CAD build for the part. Positions are in the model's coordinates, mm. A direction names the side the tool comes from. Give positions to 0.01 mm unless a question says otherwise; leave off trailing zeros. Write each loop counter-clockwise with the first axis right and the second up, starting at its lowest first coordinate (ties: lowest second). Pieces come first, ordered by that corner, then holes. Notation, with made-up numbers: (65, -25) -> (105, -25) arc R20 ccw to (105, -11) -> close; hole circle Ø3 at (-7.75, -15.75). An arc over 180 degrees is marked (long way). Answer as a JSON object with one key per item and string values.
```python
from build123d import *

# Parameters (mm, degrees)
SKETCH1_W                     = 30
SKETCH1_H                     = 30
BOSS_EXTRUDE1_DEPTH           = 30
SKETCH2_W                     = 20
SKETCH2_H                     = 20
CUT_EXTRUDE1_DEPTH            = 37.742346142
SKETCH3_W                     = 30
SKETCH3_H                     = 5
BOSS_EXTRUDE2_DEPTH           = 40
SKETCH4_R                     = 5.5
SKETCH4_R_2                   = 1.8
CUT_EXTRUDE2_DEPTH            = 65.420493634
CUT_EXTRUDE3_DEPTH            = 63.24949799
SKETCH5_W                     = 5
SKETCH5_H                     = 25
BOSS_EXTRUDE4_DEPTH           = 34
CHAMFER1_SIZE                 = 25
SKETCH8_R                     = 2.1
CUT_EXTRUDE4_DEPTH            = 63.657800791
SKETCH9_W                     = 5
SKETCH9_H                     = 30
BOSS_EXTRUDE5_DEPTH           = 12
CHAMFER2_SIZE                 = 10
CHAMFER2_SIZE2                = 5.773502692
SKETCH10_R                    = 2.1
CUT_EXTRUDE5_DEPTH            = 63.657800791
BODY_MOVE_COPY1_START         = -15
BODY_MOVE_COPY1_DEPTH         = 31
BODY_MOVE_COPY1_START_2       = -10
BODY_MOVE_COPY1_2_DEPTH       = 26
BODY_MOVE_COPY1_3_OUTLINE_W   = 34
BODY_MOVE_COPY1_3_OUTLINE_H   = 5
BODY_MOVE_COPY1_3_DEPTH       = 30
BODY_MOVE_COPY1_4_DEPTH       = 5
BODY_MOVE_COPY1_5_OUTLINE_R   = 5.5
BODY_MOVE_COPY1_5_OUTLINE_R_2 = 1.8
BODY_MOVE_COPY1_5_DEPTH       = 5
SKETCH11_W                    = 3
SKETCH11_H                    = 25
CUT_EXTRUDE6_DEPTH            = 25
SKETCH12_W                    = 25
SKETCH12_H                    = 25
CUT_EXTRUDE7_DEPTH            = 60.380131357
SKETCH13_W                    = 3
SKETCH13_H                    = 6
SKETCH13_W_2                  = 6
SKETCH13_H_2                  = 3
BOSS_EXTRUDE6_DEPTH           = 30
SKETCH14_R                    = 4.8
CUT_EXTRUDE9_DEPTH            = 2.4
CHAMFER3_SIZE                 = 12
CHAMFER3_SIZE2                = 25
FILLET1_R                     = 4
FILLET2_R                     = 4


with BuildPart() as part:
    # Sketch1 → Boss-Extrude1 (new body)
    with BuildSketch(Plane(origin=(0, 0, 0), x_dir=(1, 0, 0), z_dir=(0, 1, 0))):
        Rectangle(SKETCH1_W, SKETCH1_H)
    extrude(amount=BOSS_EXTRUDE1_DEPTH)

    # Sketch2 → Cut-Extrude1 (cut, through all)
    with BuildSketch(Plane(origin=(0, 30, 0), x_dir=(1, 0, 0), z_dir=(0, 1, 0))):
        Rectangle(SKETCH2_W, SKETCH2_H)
    extrude(amount=-CUT_EXTRUDE1_DEPTH, mode=Mode.SUBTRACT)

    # Sketch3 → Boss-Extrude2 (add)
    with BuildSketch(Plane(origin=(15, 0, 0), x_dir=(0, 0, -1), z_dir=(1, 0, 0))):
        with Locations((0, 2.5)):
            Rectangle(SKETCH3_W, SKETCH3_H)
    extrude(amount=BOSS_EXTRUDE2_DEPTH)

    # Sketch4 → Cut-Extrude2 (cut, through all)
    with BuildSketch(Plane.XZ):
        with Locations(Location((31, 0, 0), (0, 0, 270))):
            Circle(SKETCH4_R)
        with Locations(Location((19, 0, 0), (0, 0, 270))):
            Circle(SKETCH4_R_2)
        with Locations(Location((43, 0, 0), (0, 0, 270))):
            Circle(SKETCH4_R_2)
    extrude(amount=-CUT_EXTRUDE2_DEPTH, mode=Mode.SUBTRACT)

    # Sketch7 → Cut-Extrude3 (cut, through all)
    with BuildSketch(Plane(origin=(0, 5, 0), x_dir=(1, 0, 0), z_dir=(0, 1, 0))):
        Polygon((15, -15), (49, -6), (49, 15), (55, 15), (55, -15), align=None)
    extrude(amount=-CUT_EXTRUDE3_DEPTH, mode=Mode.SUBTRACT)

    # Sketch5 → Boss-Extrude4 (add)
    with BuildSketch(Plane(origin=(15, 0, 0), x_dir=(0, 0, -1), z_dir=(1, 0, 0))):
        with Locations((12.5, 17.5)):
            Rectangle(SKETCH5_W, SKETCH5_H)
    extrude(amount=BOSS_EXTRUDE4_DEPTH)

    # Chamfer1
    chamfer1_edges = [part.edges().sort_by_distance(p)[0] for p in [
        (49, 30, -12.5),
    ]]
    chamfer(chamfer1_edges, length=CHAMFER1_SIZE)

    # Sketch8 → Cut-Extrude4 (cut, through all)
    with BuildSketch(Plane.XY.offset(-10)):
        with Locations((20, 17)):
            Circle(SKETCH8_R)
    extrude(amount=-CUT_EXTRUDE4_DEPTH, mode=Mode.SUBTRACT)

    # Sketch9 → Boss-Extrude5 (add)
    with BuildSketch(Plane.ZY.offset(15)):
        with Locations((-12.5, 15)):
            Rectangle(SKETCH9_W, SKETCH9_H)
    extrude(amount=BOSS_EXTRUDE5_DEPTH)

    # Chamfer2
    chamfer2_edges = [part.edges().sort_by_distance(p)[0] for p in [
        (-27, 30, -12.5),
        (-27, 0, -12.5),
    ]]
    chamfer2_side = [part.faces().sort_by_distance(p)[0] for p in [
        (-27, 15, -12.5),
    ]]
    chamfer(chamfer2_edges, length=CHAMFER2_SIZE, length2=CHAMFER2_SIZE2, reference=chamfer2_side[0])

    # Sketch10 → Cut-Extrude5 (cut, through all)
    with BuildSketch(Plane.XY.offset(-10)):
        with Locations((-21, 17)):
            Circle(SKETCH10_R)
    extrude(amount=-CUT_EXTRUDE5_DEPTH, mode=Mode.SUBTRACT)

    # Body-Move/Copy1: read off the stored shape, not the designer's step
    # Body-Move/Copy1 outline → Body-Move/Copy1 (cut)
    with BuildSketch(Plane.XY.offset(BODY_MOVE_COPY1_START)):
        Polygon((24, 30), (21.226497308, 30), (27, 20), (27, 10), (21.226497308, 0), (49, 0), (49, 5), align=None)
        with BuildLine():
            ThreePointArc((-20.5, 14.960392195), (-17.9, 17), (-20.5, 19.039607805))
            ThreePointArc((-20.5, 19.039607805), (-18.9, 17), (-20.5, 14.960392195))
        make_face()
        with BuildLine():
            ThreePointArc((20.5, 14.960392195), (23.1, 17), (20.5, 19.039607805))
            ThreePointArc((20.5, 19.039607805), (22.1, 17), (20.5, 14.960392195))
        make_face()
    extrude(amount=BODY_MOVE_COPY1_DEPTH, mode=Mode.SUBTRACT)

    # Body-Move_Copy1 2 outline → Body-Move_Copy1 2 (cut)
    with BuildSketch(Plane.XY.offset(BODY_MOVE_COPY1_START_2)):
        Polygon((24.113248654, 5), (15, 5), (15, 0), (21.226497308, 0), align=None)
    extrude(amount=BODY_MOVE_COPY1_2_DEPTH, mode=Mode.SUBTRACT)

    # Body-Move_Copy1 3 outline → Body-Move_Copy1 3 (add)
    with BuildSketch(Plane.XY.offset(BODY_MOVE_COPY1_START)):
        with Locations((-32, 2.5)):
            Rectangle(BODY_MOVE_COPY1_3_OUTLINE_W, BODY_MOVE_COPY1_3_OUTLINE_H)
    extrude(amount=BODY_MOVE_COPY1_3_DEPTH)

    # Body-Move_Copy1 4 outline → Body-Move_Copy1 4 (add)
    with BuildSketch(Plane.XY.offset(BODY_MOVE_COPY1_START)):
        Polygon((-27, 20), (-21.226497308, 30), (-24, 30), (-49, 5), (-24.113248654, 5), (-27, 10), align=None)
        with BuildLine():
            ThreePointArc((-20.5, 14.960392195), (-22.1, 17), (-20.5, 19.039607805))
            ThreePointArc((-20.5, 19.039607805), (-23.1, 17), (-20.5, 14.960392195))
        make_face()
        with BuildLine():
            ThreePointArc((20.5, 14.960392195), (18.9, 17), (20.5, 19.039607805))
            ThreePointArc((20.5, 19.039607805), (17.9, 17), (20.5, 14.960392195))
        make_face()
    extrude(amount=BODY_MOVE_COPY1_4_DEPTH)

    # Body-Move_Copy1 5 outline → Body-Move_Copy1 5 (cut)
    with BuildSketch(Plane(origin=(0, 0, 0), x_dir=(1, 0, 0), z_dir=(0, 1, 0))):
        with Locations((-31, 0)):
            Circle(BODY_MOVE_COPY1_5_OUTLINE_R)
        with Locations((-19, 0)):
            Circle(BODY_MOVE_COPY1_5_OUTLINE_R_2)
        with Locations((-43, 0)):
            Circle(BODY_MOVE_COPY1_5_OUTLINE_R_2)
        Polygon((-49, -15), (-15, -15), (-49, -6), align=None)
    extrude(amount=BODY_MOVE_COPY1_5_DEPTH, mode=Mode.SUBTRACT)

    # Sketch11 → Cut-Extrude6 (cut)
    with BuildSketch(Plane(origin=(0, 30, 0), x_dir=(1, 0, 0), z_dir=(0, 1, 0))):
        with Locations((-13.5, -2.5)):
            Rectangle(SKETCH11_W, SKETCH11_H)
    extrude(amount=-CUT_EXTRUDE6_DEPTH, mode=Mode.SUBTRACT)

    # Sketch12 → Cut-Extrude7 (cut, through all)
    with BuildSketch(Plane(origin=(0, 30, 0), x_dir=(1, 0, 0), z_dir=(0, 1, 0))):
        with Locations((2.5, -2.5)):
            Rectangle(SKETCH12_W, SKETCH12_H)
    extrude(amount=-CUT_EXTRUDE7_DEPTH, mode=Mode.SUBTRACT)

    # Sketch13 → Boss-Extrude6 (add)
    with BuildSketch(Plane(origin=(0, 30, 0), x_dir=(1, 0, 0), z_dir=(0, 1, 0))):
        with Locations((-8.5, 0)):
            Rectangle(SKETCH13_W, SKETCH13_H)
        with Locations((0, 8.5)):
            Rectangle(SKETCH13_W_2, SKETCH13_H_2)
    extrude(amount=-BOSS_EXTRUDE6_DEPTH)

    # Sketch14 → Cut-Extrude9 (cut)
    with BuildSketch(Plane.XY.offset(-10)):
        with Locations((-20, 17)):
            Circle(SKETCH14_R)
        with Locations((21, 17)):
            Circle(SKETCH14_R)
    extrude(amount=-CUT_EXTRUDE9_DEPTH, mode=Mode.SUBTRACT)

    # Chamfer3
    chamfer3_edges = [part.edges().sort_by_distance(p)[0] for p in [
        (-11, 30, 15),
    ]]
    chamfer3_side = [part.faces().sort_by_distance(p)[0] for p in [
        (-18, 30, -10.542718717),
    ]]
    chamfer(chamfer3_edges, length=CHAMFER3_SIZE, length2=CHAMFER3_SIZE2, reference=chamfer3_side[0])

    # Fillet1
    fillet1_edges = [part.edges().sort_by_distance(p)[0] for p in [
        (-49, 2.5, 6),
        (-15, 2.5, 15),
    ]]
    fillet(fillet1_edges, radius=FILLET1_R)

    # Fillet2
    fillet2_edges = [part.edges().sort_by_distance(p)[0] for p in [
        (27, 10, -12.5),
        (27, 20, -12.5),
        (21.226497308, 30, -12.5),
        (-24, 30, -12.5),
    ]]
    fillet(fillet2_edges, radius=FILLET2_R)


solid = part.part
```
1) Mould opens along X. For faces 1 (the flat face through (3, 15, -8)), 2 (the cylindrical face through (20.38, 21.76, -11.18)), 3 (the flat face through (-37, 17, -13)) say: released by +X, released by -X, zero draft, split by the parting line, or undercut.
Model answer:
{"face 1": "released by +X", "face 2": "undercut", "face 3": "released by -X"}
2) Pin check, flat tips, straight feed: pin 1 (5 mm diameter, centred on x = -27, z = -10, fed in from +Y); pin 2 (12.5 mm diameter, centred on x = -39, z = -0.5, fed in from +Y); pin 3 (3.5 mm diameter, centred on x = -7, y = 12.5, fed in from +Z); pin 4 (2.5 mm diameter, centred on x = 21, y = 17, fed in from -Z). Stop position of each tip, or through.
Model answer:
{"pin 1": "stops at y = 29.37", "pin 2": "stops at y = 5", "pin 3": "stops at z = 3", "pin 4": "passes through"}
3) Slice it at A-A (y = 17). State how many separate pieces and enclosed holes the cut face has, then the cut area to 3 significant figures.
Model answer:
{"separate pieces": "3", "enclosed holes": "0", "area": "327 mm2"}
4) Wall check: probe 1 along X at (y, z) = (2.1, 0); probe 2 along X at (y, z) = (17, -14.5); probe 3 along X at (y, z) = (22.75, -9.5). Give the ranges that are in metal, low to high.
Model answer:
{"probe 1": "x = -49 to -44.8, -41.2 to -36.5, -25.5 to -20.8, -17.2 to -7", "probe 2": "x = -37 to -22.1, -17.9 to 18.9, 23.1 to 27", "probe 3": "x = -12 to -10, -3 to 3"}
5) Slice it at C-C (x = -32). List the corners of the cut face in (y, z), then the cut area to 3 significant figures.
Model answer:
{"outline": "(0, -15) -> (22, -15) -> (22, -10) -> (5, -10) -> (5, -5.41) -> (0, -5.41) -> close; (0, 5.41) -> (5, 5.41) -> (5, 10.5) -> (0, 10.5) -> close", "area": "158 mm2"}
6) Slice it at B-B (z = 0). List the corners of the cut face in (x, y), then the cut area to 3 significant figures.
Model answer:
{"outline": "(-49, 0) -> (-44.8, 0) -> (-44.8, 5) -> (-49, 5) -> close; (-41.2, 0) -> (-36.5, 0) -> (-36.5, 5) -> (-41.2, 5) -> close; (-25.5, 0) -> (-20.8, 0) -> (-20.8, 5) -> (-25.5, 5) -> close; (-17.2, 0) -> (-7, 0) -> (-7, 30) -> (-12, 30) -> (-12, 5) -> (-17.2, 5) -> close", "area": "244 mm2"}
7) 3-axis set-ups, long thin cutter, end or side, ignore diameter. For faces 4 (the flat face through (-10, 9, 8)), 5 (the flat face through (-7, 15, -10)), 6 (the flat face through (-3, 15, -8)), 7 (the flat face through (-9, 15, -3)), 8 (the flat face through (-19, 14.9, -12.4)): which of +Z, -Z, +X, -X, +Y, -Y reach the whole face in a straight line?
Model answer:
{"face 4": "+Z, +X, +Y, -Y", "face 5": "+Y, -Y", "face 6": "+Z, +Y, -Y", "face 7": "+X, +Y, -Y", "face 8": "+Z"}
8) Slice it at D-D (z = -11). List the corners of the cut face in (x, y), then the cut area to 3 significant figures.
Model answer:
{"outline": "(-49, 0) -> (21.23, 0) -> (26.46, 9.07) arc R4 ccw to (27, 11.07) -> (27, 18.93) arc R4 ccw to (26.46, 20.93) -> (22.38, 28) arc R4 ccw to (18.92, 30) -> (-22.34, 30) arc R4 ccw to (-25.17, 28.83) -> (-49, 5) -> close; hole circle Ø9.6 at (-20, 17); hole circle Ø9.6 at (21, 17)", "area": "1,760 mm2"}
